Verification items for the finished model (mm, model axes). A direction names the side the tool comes from. Give positions to 0.01 mm unless a question says otherwise; leave off trailing zeros. Write each loop counter-clockwise with the first axis right and the second up, starting at its lowest first coordinate (ties: lowest second). Pieces come first, ordered by that corner, then holes. Notation, with made-up numbers: (-30, 8) -> (27, 8) arc R18 cw to (27, 33) -> close; hole circle Ø10 at (9.25, -5.75). An arc over 180 degrees is marked (long way). Use one line per item in the form item = value. Start each with the question number.
(1) Section check D-D, the plane x = -4. Record the cut outline in (y, z), plus the area to 3 significant figures.
(2) Section check A-A, the plane y = 0. Record the cut outline in (x, z), plus the area to 3 significant figures.
(3) Scan lines: L1, parallel to Z at x = -4.75, y = 2.5; L2, parallel to X at y = 0.25, z = 19.75; L3, parallel to X at y = 1.75, z = 16.75. Record each from-to range of solid material in increasing order.
(4) Section check B-B, the plane z = 17. Record the cut outline in (x, y), plus the area to 3 significant figures.
(5) Set-up check for faces 1 (the face through (-4.73, 3.85, 13.9)), 2 (the face through (0, 2, 14)), 3 (the face through (-2, -5, 6.5)): record each of +Z, -Z, +X, -X, +Y, -Y from which the full face is reachable in a straight line by a thin tool's end or side.
(6) Depth check by flat-ended pin: pin 1 Ø0.7 at (x, y) = (1, 1.5) entering from -Z; pin 2 Ø1.5 at (x, z) = (-0.5, 17.5) entering from -Y; pin 3 Ø3 at (y, z) = (0.5, 10.5) entering from +X; pin 4 Ø3 at (x, y) = (-2, -1) entering from -Z. Enter the tip coordinate at first touch or a pass-through.
(7) Section check C-C, the plane x = 0. Record the cut outline in (y, z), plus the area to 3 significant figures.
Autodesk Fusion 360 part; units mm, degrees
sketch "Skizze1" plane through (0, 0, 0) normal (0, 0, 1) x (1, 0, 0)
  line L0 (1.95, -2.0094) -> (-1.95, 2.0094) construction
  line L1 (-1.95, 2.0094) -> (1.95, 2.0094)
  circle A0 centre (0, 0) radius 5
  line L2 (1.95, 2.0094) -> (1.95, -2.0094)
  line L3 (-1.95, -2.0094) -> (1.95, 2.0094) construction
  circle A1 centre (0, 0) radius 2.8
  line L4 (-1.95, -2.0094) -> (-1.95, 2.0094)
  line L5 (1.95, -2.0094) -> (-1.95, -2.0094)
  dimension "d1" = 5.6
  dimension "d2" = 10
  dimension "d3" = 3.9
extrude "Extrusion1" add sketch "Skizze1" along normal blind 6.5 contours A1 L4 | L2 A1 | A0
sketch "Skizze2" plane through (0, 0, 6.5) normal (0, 0, 1) x (-1, 0, 0)
  arc A0 (-1.95, -2.0094) -> (1.95, -2.0094) centre (0, 0) ccw
  line L0 (-1.95, -2.0094) -> (-1.95, 2.0094)
  arc A1 (1.95, 2.0094) -> (-1.95, 2.0094) centre (0, 0) ccw
  line L1 (1.95, 2.0094) -> (1.95, -2.0094)
  circle A2 centre (0, 0) radius 5
  line L2 (-6.9634, 1.0605) -> (-4.4001, -5.5002)
  line L3 (-4.4001, -5.5002) -> (2.5632, -6.5607)
  line L4 (2.5632, -6.5607) -> (6.9634, -1.0605)
  line L5 (6.9634, -1.0605) -> (4.4001, 5.5002)
  line L6 (4.4001, 5.5002) -> (-2.5632, 6.5607)
  line L7 (-2.5632, 6.5607) -> (-6.9634, 1.0605)
  circle A3 centre (0, 0) radius 2
  dimension "d6" = 6.1
  dimension "d9" = 4
extrude "Extrusion2" add sketch "Skizze2" along normal blind 15 contours L0 A3 | L1 A3 | A2 | L2 L3 L4 L5 L6 L7
extrude "Extrusion3" add sketch "Skizze2" along normal blind 15 contours A0 L0 L1 A3 | L0 A1 L1 A3 | A2
Completed:
q1.outline = (-5.56, 6.5) -> (-3, 6.5) -> (-3, 0) -> (3, 0) -> (3, 6.5) -> (4.76, 6.5) -> (4.76, 21.5) -> (-5.56, 21.5) -> close
q1.area = 194 mm²
q2.outline = (-6.55, 6.5) -> (-5, 6.5) -> (-5, 0) -> (-1.95, 0) -> (-1.95, 21.5) -> (-6.55, 21.5) -> close; (1.95, 0) -> (5, 0) -> (5, 6.5) -> (6.55, 6.5) -> (6.55, 21.5) -> (1.95, 21.5) -> close
q2.area = 178 mm²
q3.L1 = 6.5 to 21.5
q3.L2 = -6.65 to -1.95, 1.95 to 6.45
q3.L3 = -6.41 to -0.97, 0.97 to 5.87
q4.outline = (-6.96, 1.06) -> (-4.4, -5.5) -> (2.56, -6.56) -> (6.96, -1.06) -> (4.4, 5.5) -> (-2.56, 6.56) -> close; hole (-1.95, -0.44) arc R2 ccw to (1.95, -0.44) -> (1.95, 0.44) arc R2 ccw to (-1.95, 0.44) -> close
q4.area = 116 mm²
q5.face_1 = +Z, -Z, -X, +Y
q5.face_2 = +Z, -Z
q5.face_3 = -Z
q6.pin_1 = 6.5
q6.pin_2 = -6.21
q6.pin_3 = 6.94
q6.pin_4 = 0
q7.outline = (-6.17, 6.5) -> (-5, 6.5) -> (-5, 0) -> (-2.8, 0) -> (-2.8, 6.5) -> (-2, 6.5) -> (-2, 21.5) -> (-6.17, 21.5) -> close; (2, 6.5) -> (2.8, 6.5) -> (2.8, 0) -> (5, 0) -> (5, 6.5) -> (6.17, 6.5) -> (6.17, 21.5) -> (2, 21.5) -> close
q7.area = 154 mm²
